from build123d import *

# Parameters (mm, degrees)
SKETCH_1_R      = 14.4
SKETCH_1_R_2    = 8.6
EXTRUDE_1_DEPTH = 80
EXTRUDE_START   = 3
SKETCH_1_3_R    = 19
SKETCH_1_3_R_2  = 16
SKETCH_1_3_R_3  = 14.4
SKETCH_1_3_R_4  = 8.6
EXTRUDE_2_DEPTH = 3
SKETCH_1_5_R    = 19
SKETCH_1_5_R_2  = 16
EXTRUDE_3_DEPTH = 30
EXTRUDE_START_2 = -77
SKETCH_1_6_R    = 8.6
EXTRUDE_4_DEPTH = 3


with BuildPart() as part:
    # Эскиз1 → Бобышка-Вытянуть1 (new body)
    with BuildSketch(Plane.XY):
        Circle(SKETCH_1_R)
        Circle(SKETCH_1_R_2, mode=Mode.SUBTRACT)
    extrude(amount=-EXTRUDE_1_DEPTH)

    # Эскиз1<3> → Бобышка-Вытянуть2 (add)
    # profile 1 of 3: a face of its own
    with BuildSketch(Plane.XY.offset(EXTRUDE_START)):
        Circle(SKETCH_1_3_R)
        Circle(SKETCH_1_3_R_2, mode=Mode.SUBTRACT)
    # profile 2 of 3: a face of its own
    with BuildSketch(Plane.XY.offset(EXTRUDE_START)):
        Circle(SKETCH_1_3_R_2)
        Circle(SKETCH_1_3_R_3, mode=Mode.SUBTRACT)
    # profile 3 of 3: a face of its own
    with BuildSketch(Plane.XY.offset(EXTRUDE_START)):
        Circle(SKETCH_1_3_R_3)
        Circle(SKETCH_1_3_R_4, mode=Mode.SUBTRACT)
    extrude(amount=-EXTRUDE_2_DEPTH)

    # Эскиз1<5> → Бобышка-Вытянуть3 (add)
    with BuildSketch(Plane.XY):
        Circle(SKETCH_1_5_R)
        Circle(SKETCH_1_5_R_2, mode=Mode.SUBTRACT)
    extrude(amount=-EXTRUDE_3_DEPTH)

    # Эскиз1<6> → Бобышка-Вытянуть4 (add)
    with BuildSketch(Plane.XY.offset(EXTRUDE_START_2)):
        Circle(SKETCH_1_6_R)
    extrude(amount=-EXTRUDE_4_DEPTH)


solid = part.part
Verification items for the finished model (mm, model axes). A direction names the side the tool comes from. Coordinates: 2 decimals unless noted, no trailing zeros. Order: outer loops, then holes, each group sorted by start corner. A loop starts at its lowest first (then second) coordinate and runs counter-clockwise, first axis right, second up. Notation, with made-up numbers: M 83.5,47.25 L 92.5,47.25 A26 ccw 92.5,75.25 Z; hole C -28.5,-19 d7. An arc over 180 degrees is marked long. Return JSON: item names as keys, results as strings.
1) Cross-section at D-D, the plane z = -69.5. Record the boundary of the cut face in (x, y), and give its area (3 significant figures).
Answer list:
{"outline": "C 0,0 d28.8; hole C 0,0 d17.2", "area": "419 mm2"}
2) Thickness scan on L1, parallel to Y at x = 0, z = -56.5; L2, parallel to Y at x = -3, z = -13; L3, parallel to Z at x = -16.5, y = -7. Record the ranges inside material, lowest first. Write a range as [from, to].
Answer list:
{"L1": "[-14.4, -8.6], [8.6, 14.4]", "L2": "[-18.76, -15.72], [-14.08, -8.06], [8.06, 14.08], [15.72, 18.76]", "L3": "[-30, 3]"}
3) Access from +Z, -Z, +X, -X, +Y, -Y to the whole of each face (thin tool, end or side, straight path). Record for faces 4 (the cylindrical face through (-3.47, -15.62, -14.79)), 5 (the cylindrical face through (-8.59, 0.38, -36.44)), 6 (the flat face through (0, 0, -80)).
Answer list:
{"face 4": "-Z", "face 5": "+Z", "face 6": "-Z, +X, -X, +Y, -Y"}
4) Gauge pin test, flat ends, axial feed: pin 1 (6 mm diameter, centred on y = -9.5, z = -34, fed in from -X); pin 2 (12 mm diameter, centred on x = 7, z = -23, fed in from -Y); pin 3 (5 mm diameter, centred on x = 4.5, z = -36.5, fed in from -Y). Record the tip position at first contact, or that the pin passes through.
Answer list:
{"pin 1": "x = -12.85", "pin 2": "y = -18.97", "pin 3": "y = -14.26"}
5) Cross-section at B-B, the plane x = 0. Record the boundary of the cut face in (y, z), and give its area (3 significant figures).
Answer list:
{"outline": "M -19,-30 L -16,-30 L -16,0 L -14.4,0 L -14.4,-80 L 14.4,-80 L 14.4,0 L 16,0 L 16,-30 L 19,-30 L 19,3 L 8.6,3 L 8.6,-77 L -8.6,-77 L -8.6,3 L -19,3 Z", "area": "1,220 mm2"}
6) Cross-section at A-A, the plane z = -27. Record the boundary of the cut face in (x, y).
Answer list:
{"outline": "C 0,0 d38; C 0,0 d28.8; hole C 0,0 d32; hole C 0,0 d17.2"}
7) Release check for a two-part mould opening along X. For faces 1 (the flat face through (0, 0, -77)), 2 (the cylindrical face through (8.767, -16.856, -13.269)), 3 (the flat face through (-10, -13, -30)) record: +X half, -X half, draft (parallel to the pull), parting line (faces both ways), or undercut.
Answer list:
{"face 1": "undercut", "face 2": "parting line", "face 3": "draft"}
